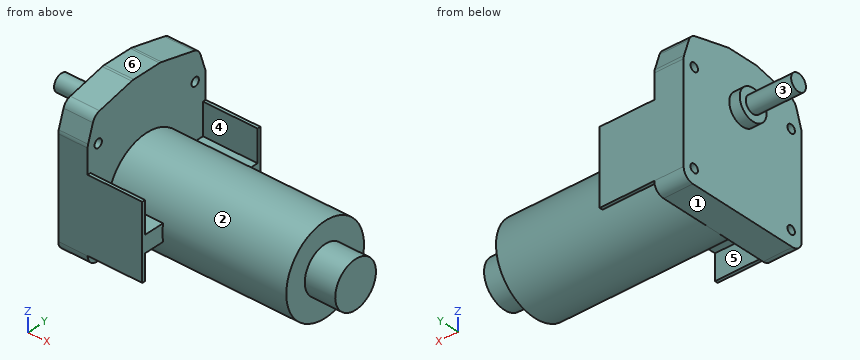
```python
from build123d import *

# Parameters (mm, degrees)
ESQUISSE1_R       = 2
EXTRUSION3_DEPTH  = 14
ESQUISSE3_R       = 21
EXTRUSION4_DEPTH  = 85
ESQUISSE4_R       = 4
EXTRUSION5_DEPTH  = 26.6
ESQUISSE5_R       = 7.25
EXTRUSION6_DEPTH  = 5
EXTRUSION9_DEPTH  = 26
ESQUISSE9_R       = 11
EXTRUSION10_DEPTH = 14.5


with BuildPart() as part:
    # Esquisse1 → Extrusion3 (new body)
    with BuildSketch(Plane(origin=(0, 0, 0), x_dir=(0, 0, -1), z_dir=(1, 0, 0))):
        with BuildLine():
            Line((-6, 31.9), (40.5, 31.9))
            ThreePointArc((40.5, 31.9), (44.035533906, 30.435533906), (45.5, 26.9))
            Line((45.5, 26.9), (45.5, -26.9))
            ThreePointArc((45.5, -26.9), (44.035533906, -30.435533906), (40.5, -31.9))
            Line((40.5, -31.9), (-6, -31.9))
            ThreePointArc((-6, -31.9), (-6.782039696, -31.838462708), (-7.54482955, -31.655365566))
            Line((-7.54482955, -31.655365566), (-15.54482955, -29.056483056))
            ThreePointArc((-15.54482955, -29.056483056), (-17.685916108, -27.679581999), (-18.871597264, -25.426968324))
            Line((-18.871597264, -25.426968324), (-22.871597264, -8.118823709))
            ThreePointArc((-22.871597264, -8.118823709), (-22.967795604, -7.559547531), (-23, -6.992972875))
            Line((-23, -6.992972875), (-23, 6.992972875))
            ThreePointArc((-23, 6.992972875), (-22.967795604, 7.559547531), (-22.871597264, 8.118823709))
            Line((-22.871597264, 8.118823709), (-18.871597264, 25.426968324))
            ThreePointArc((-18.871597264, 25.426968324), (-17.685916108, 27.679581999), (-15.54482955, 29.056483056))
            Line((-15.54482955, 29.056483056), (-7.54482955, 31.655365566))
            ThreePointArc((-7.54482955, 31.655365566), (-6.782039696, 31.838462708), (-6, 31.9))
        make_face()
        with Locations((38.44, -26.2)):
            Circle(ESQUISSE1_R, mode=Mode.SUBTRACT)
        with Locations((-5.16, -26.2)):
            Circle(ESQUISSE1_R, mode=Mode.SUBTRACT)
        with Locations((-5.16, 26.2)):
            Circle(ESQUISSE1_R, mode=Mode.SUBTRACT)
        with Locations((38.44, 26.2)):
            Circle(ESQUISSE1_R, mode=Mode.SUBTRACT)
    extrude(amount=EXTRUSION3_DEPTH)

    # Esquisse3 → Extrusion4 (add)
    with BuildSketch(Plane(origin=(14, 0, 0), x_dir=(0, 0, -1), z_dir=(1, 0, 0))):
        with Locations((24.5, 0)):
            Circle(ESQUISSE3_R)
    extrude(amount=EXTRUSION4_DEPTH)

    # Esquisse4 → Extrusion5 (add)
    with BuildSketch(Plane(origin=(0, 0, 0), x_dir=(0, 0, -1), z_dir=(1, 0, 0))):
        Circle(ESQUISSE4_R)
    extrude(amount=-EXTRUSION5_DEPTH)

    # Esquisse5 → Extrusion6 (add)
    with BuildSketch(Plane(origin=(0, 0, 0), x_dir=(0, 0, -1), z_dir=(1, 0, 0))):
        Circle(ESQUISSE5_R)
    extrude(amount=-EXTRUSION6_DEPTH)

    # Esquisse8 → Extrusion9 (add)
    with BuildSketch(Plane(origin=(14, 0, 0), x_dir=(0, 0, -1), z_dir=(1, 0, 0))):
        Polygon((40.5, 31.9), (5.5, 31.9), (5.5, 30.4), (20.5, 30.4), (20.5, 13.147221685), (28.5, 13.147221685), (28.5, 30.4), (40.5, 30.4), align=None)
        Polygon((40.5, -30.4), (40.5, -31.9), (5.5, -31.9), (5.5, -30.4), (20.5, -30.4), (20.5, -13.147221685), (28.5, -13.147221685), (28.5, -30.4), align=None)
    extrude(amount=EXTRUSION9_DEPTH)

    # Esquisse9 → Extrusion10 (add)
    with BuildSketch(Plane(origin=(99, 0, 0), x_dir=(0, 0, -1), z_dir=(1, 0, 0))):
        with Locations((24.5, 0)):
            Circle(ESQUISSE9_R)
    extrude(amount=EXTRUSION10_DEPTH)


solid = part.part
```
Part model, mm, in its own coordinate system. Face numbers are marked on the shaded views. A direction names the side the tool comes from. Round coordinates to 2 decimals unless told otherwise and drop trailing zeros. Loops run counter-clockwise (first coordinate to the right, second up) from the corner with the lowest first, then second, coordinate; pieces in that order, holes last.
Item 1: Cut at B-B, the plane x = 17. Give the cut face in (y, z).
Item 2: Cut at A-A, the plane z = 0. Give the cut face in (x, y), then the cut area to 3 significant figures.
Item 3: 3-axis set-ups, long thin cutter, end or side, ignore diameter. For the marked faces 1 and 2: which of +Z, -Z, +X, -X, +Y, -Y reach the whole face in a straight line?
Item 4: Drop flat-ended pins along their axis: P1, Ø5, axis at y = 10.5, z = 10.5, coming from the +X side; P2, Ø10, axis at x = 78.5, z = -15, coming from the -Y side; P3, Ø12, axis at y = 14.5, z = -16, coming from the -X side. Give the stop position or say it passes through.
Item 5: Cut at D-D, the plane y = -14.5. Give the cut face in (x, z).
Item 6: Drill centre lines: line 1 (Y direction, x = 6.5, z = -38.44); line 2 (Z direction, x = 26.5, y = 28.5); line 3 (X direction, y = 15, z = -36.5). Where is each one in solid material? Low to high.
Item 7: Mould opens along Y. For the marked faces 3, 4, 5 and 6 say: +Y half, -Y half, draft (parallel to the pull), parting line (faces both ways), or undercut.
Item 8: Cut at C-C, the plane x = 1.5. Give the cut face in (y, z).
A:
1. outline: (-31.9, -40.5) - (-30.4, -40.5) - (-30.4, -28.5) - (-20.62, -28.5) arc R21 ccw to (20.62, -28.5) - (30.4, -28.5) - (30.4, -40.5) - (31.9, -40.5) - (31.9, -5.5) - (30.4, -5.5) - (30.4, -20.5) - (20.62, -20.5) arc R21 ccw to (-20.62, -20.5) - (-30.4, -20.5) - (-30.4, -5.5) - (-31.9, -5.5) - close
2. outline: (-26.6, -4) - (-5, -4) - (-5, -7.25) - (0, -7.25) - (0, -31.9) - (14, -31.9) - (14, 31.9) - (0, 31.9) - (0, 7.25) - (-5, 7.25) - (-5, 4) - (-26.6, 4) - close
2. area: 1,140 mm2
3. face 1: -Z, +X, -X, +Y, -Y
3. face 2: +X
4. P1: stops at x = 14
4. P2: stops at y = -20.51
4. P3: stops at x = 0
5. outline: (0, -45.5) - (14, -45.5) - (14, -39.69) - (99, -39.69) - (99, -9.31) - (14, -9.31) - (14, 21.4) - (0, 21.4) - close
6. line 1: y = -31.9 to -28.2, -24.2 to 24.2, 28.2 to 31.9
6. line 2: z = -28.5 to -20.5
6. line 3: x = 0 to 99
7. face 3: parting line
7. face 4: undercut
7. face 5: undercut
7. face 6: draft
8. outline: (-31.9, -40.5) arc R5 ccw to (-26.9, -45.5) - (26.9, -45.5) arc R5 ccw to (31.9, -40.5) - (31.9, 6) arc R5 ccw to (31.66, 7.54) - (29.06, 15.54) arc R5 ccw to (25.43, 18.87) - (8.12, 22.87) arc R5 ccw to (6.99, 23) - (-6.99, 23) arc R5 ccw to (-8.12, 22.87) - (-25.43, 18.87) arc R5 ccw to (-29.06, 15.54) - (-31.66, 7.54) arc R5 ccw to (-31.9, 6) - close; hole circle Ø4 at (-26.2, -38.44); hole circle Ø4 at (-26.2, 5.16); hole circle Ø4 at (26.2, -38.44); hole circle Ø4 at (26.2, 5.16)
